```python
from build123d import *

# Parameters (mm, degrees)
F0_R     = 15
F0_R_2   = 7.5
F1_DEPTH = 9
F2_SIZE  = 0.5
F3_R     = 8
F3_R_2   = 7.5
F4_DEPTH = 0.1


with BuildPart() as f1:
    # F0 (on Front) → F1 (new body)
    with BuildSketch(Plane.XZ):
        Circle(F0_R)
        Circle(F0_R_2, mode=Mode.SUBTRACT)
    extrude(amount=F1_DEPTH)

    # F2
    f2_edges = [f1.edges().sort_by_distance(p)[0] for p in [
        (-15, -9, 0),
        (15, -4.5, 0),
        (-15, 0, 0),
    ]]
    chamfer(f2_edges, length=F2_SIZE)

    # F3 (on face) → F4 (join)
    with BuildSketch(Plane.XZ.offset(9)):
        Circle(F3_R)
        Circle(F3_R_2, mode=Mode.SUBTRACT)
    extrude(amount=F4_DEPTH)


solid = f1.part
```
Build history of the part. All positions in model axes, mm. A direction names the side the tool comes from. Coordinates: 2 decimals unless noted, no trailing zeros. Write each loop counter-clockwise with the first axis right and the second up, starting at its lowest first coordinate (ties: lowest second). Pieces come first, ordered by that corner, then holes.
1. Drop a flat-ended pin along its axis: pin 1 (1 mm diameter, centred on y = -2, z = -11.5, fed in from -X). Give the stop position or say it passes through.
Answer block:
pin 1: stops at x = -10.2
2. Band-saw the part on C-C, the plane y = -8. Give the cut face in (x, z), and give its area (3 significant figures).
Answer block:
outline: circle Ø30 at (0, 0); hole circle Ø15 at (0, 0)
area: 530 mm2
3. Band-saw the part on B-B, the plane x = 0. Give the cut face in (y, z), and give its area (3 significant figures).
Answer block:
outline: (-9.1, -8) - (-9, -8) - (-9, -14.5) - (-8.5, -15) - (-0.5, -15) - (0, -14.5) - (0, -7.5) - (-9.1, -7.5) - close; (-9.1, 7.5) - (0, 7.5) - (0, 14.5) - (-0.5, 15) - (-8.5, 15) - (-9, 14.5) - (-9, 8) - (-9.1, 8) - close
area: 135 mm2
4. 3-axis set-ups, long thin cutter, end or side, ignore diameter. For faces 1 (the flat face through (6, -9, -6)), 2 (the cylindrical face through (-7.493, -4.486, 0.33)): which of +Z, -Z, +X, -X, +Y, -Y reach the whole face in a straight line?
Answer block:
face 1: -Y
face 2: +Y, -Y
5. Drill centre lines: probe 1 along Z at (x, y) = (0, -3.5); probe 2 along X at (y, z) = (-2.25, 4.5); probe 3 along Y at (x, z) = (-13, -6.25). Where is each one in solid material? Low to high.
Answer block:
probe 1: z = -15 to -7.5, 7.5 to 15
probe 2: x = -14.31 to -6, 6 to 14.31
probe 3: y = -9 to 0
6. Band-saw the part on A-A, the plane z = 0. Give the cut face in (x, y).
Answer block:
outline: (-15, -8.5) - (-14.5, -9) - (-8, -9) - (-8, -9.1) - (-7.5, -9.1) - (-7.5, 0) - (-14.5, 0) - (-15, -0.5) - close; (7.5, -9.1) - (8, -9.1) - (8, -9) - (14.5, -9) - (15, -8.5) - (15, -0.5) - (14.5, 0) - (7.5, 0) - close
